Geometry check sheet. Reference: the model listing, model coordinates, mm. Face numbers are marked on the shaded views. A direction names the side the tool comes from. Round coordinates to 2 decimals unless told otherwise and drop trailing zeros. Write each loop counter-clockwise with the first axis right and the second up, starting at its lowest first coordinate (ties: lowest second). Pieces come first, ordered by that corner, then holes. Notation, with made-up numbers: (59, 5.5) - (79, 5.5) arc R24 cw to (79, 25.5) - close; hole circle Ø4 at (0.5, 8.5). An arc over 180 degrees is marked (long way). Return JSON: item names as keys, results as strings. Group by question number.
from build123d import *

# Parameters (mm, degrees)
SKETCH_2_R          = 1.5
EXTRUDE_1_DEPTH     = 27
SHELL_1_DEPTH       = 24
CUT_EXTRUDE_START   = -24
SKETCH_3_R          = 3
CUT_EXTRUDE_1_DEPTH = 24
SKETCH_5_W          = 20
SKETCH_5_H          = 6
CUT_EXTRUDE_3_DEPTH = 32
SKETCH_6_W          = 4
SKETCH_6_H          = 12
CUT_EXTRUDE_4_DEPTH = 32
SKETCH_7_W          = 10
SKETCH_7_H          = 8
CUT_EXTRUDE_5_DEPTH = 32
EXTRUDE_2_DEPTH     = 24
SKETCH_9_W          = 10
SKETCH_9_H          = 3
CUT_EXTRUDE_6_DEPTH = 24
SKETCH_10_R         = 1.35
CUT_EXTRUDE_7_DEPTH = 10
CUT_EXTRUDE_8_DEPTH = 10


# Read off the part's stored shape, not the designer's step: 抽壳1
with BuildPart() as part:
    # 草图2 → 凸台-拉伸1 (new body)
    with BuildSketch(Plane.XY):
        with BuildLine():
            Line((-76.5, 30.151923789), (-76.5, -30.151923789))
            ThreePointArc((-76.5, -30.151923789), (-77.380060021, -34.576284287), (-72.878679656, -34.871320344))
            Line((-72.878679656, -34.871320344), (-57.32, -50.43))
            Line((-57.32, -50.43), (57.32, -50.43))
            Line((57.32, -50.43), (72.878679656, -34.871320344))
            ThreePointArc((72.878679656, -34.871320344), (77.380060021, -34.576284287), (76.5, -30.151923789))
            Line((76.5, -30.151923789), (76.5, 30.151923789))
            ThreePointArc((76.5, 30.151923789), (77.593259199, 34.258312544), (73.483390382, 35.33841559))
            Line((73.483390382, 35.33841559), (40.238526366, 54.25))
            Line((40.238526366, 54.25), (-40.760907637, 54.25))
            Line((-40.760907637, 54.25), (-73.5, 35.348076211))
            ThreePointArc((-73.5, 35.348076211), (-77.598076211, 34.25), (-76.5, 30.151923789))
        make_face()
        with Locations((-75, 32.75)):
            Circle(SKETCH_2_R, mode=Mode.SUBTRACT)
        with Locations((75, 32.75)):
            Circle(SKETCH_2_R, mode=Mode.SUBTRACT)
        with Locations((75, -32.75)):
            Circle(SKETCH_2_R, mode=Mode.SUBTRACT)
        with Locations((-75, -32.75)):
            Circle(SKETCH_2_R, mode=Mode.SUBTRACT)
    extrude(amount=EXTRUDE_1_DEPTH)

    # 抽壳1 outline → 抽壳1 (cut)
    with BuildSketch(Plane.XY):
        with BuildLine():
            Line((-73.5, 28.507359313), (-73.5, -28.507359313))
            ThreePointArc((-73.5, -28.507359313), (-71.254879923, -30.255190266), (-70.506971411, -33.000387902))
            Line((-70.506971411, -33.000387902), (-56.077359313, -47.43))
            Line((-56.077359313, -47.43), (56.077359313, -47.43))
            Line((56.077359313, -47.43), (70.506971411, -33.000387902))
            ThreePointArc((70.506971411, -33.000387902), (71.254879923, -30.255190266), (73.5, -28.507359313))
            Line((73.5, -28.507359313), (73.5, 28.507359313))
            ThreePointArc((73.5, 28.507359313), (71.110106029, 30.48754008), (70.570593139, 33.543948905))
            Line((70.570593139, 33.543948905), (39.444948236, 51.25))
            Line((39.444948236, 51.25), (-39.95706006, 51.25))
            Line((-39.95706006, 51.25), (-70.575765386, 33.572282238))
            ThreePointArc((-70.575765386, 33.572282238), (-71.102885683, 30.5), (-73.5, 28.507359313))
        make_face()
    extrude(amount=SHELL_1_DEPTH, mode=Mode.SUBTRACT)

    # 草图3 → 切除-拉伸1 (cut)
    with BuildSketch(Plane.XY.offset(27).offset(CUT_EXTRUDE_START)):
        with Locations((75, 32.75)):
            Circle(SKETCH_3_R)
        with Locations((75, -32.75)):
            Circle(SKETCH_3_R)
        with Locations((-75, -32.75)):
            Circle(SKETCH_3_R)
        with Locations((-75, 32.75)):
            Circle(SKETCH_3_R)
    extrude(amount=CUT_EXTRUDE_1_DEPTH, mode=Mode.SUBTRACT)

    # 草图5 → 切除-拉伸3 (cut)
    with BuildSketch(Plane.XY.offset(27)):
        with Locations((20.7074416, -19.577067137)):
            Rectangle(SKETCH_5_W, SKETCH_5_H)
    extrude(amount=-CUT_EXTRUDE_3_DEPTH, mode=Mode.SUBTRACT)

    # 草图6 → 切除-拉伸4 (cut)
    with BuildSketch(Plane(origin=(76.5, 0, 0), x_dir=(0, 0, -1), z_dir=(1, 0, 0))):
        with Locations((-2, 20.977362477)):
            Rectangle(SKETCH_6_W, SKETCH_6_H)
    extrude(amount=-CUT_EXTRUDE_4_DEPTH, mode=Mode.SUBTRACT)

    # 草图7 → 切除-拉伸5 (cut)
    with BuildSketch(Plane(origin=(33.153284591, 58.280491682, 0), x_dir=(0.8692042501767389, -0.4944532045347601, 0), z_dir=(0.4944532045347601, 0.8692042501767389, 0))):
        with Locations((38.03253292, -4)):
            Rectangle(SKETCH_7_W, SKETCH_7_H)
    extrude(amount=-CUT_EXTRUDE_5_DEPTH, mode=Mode.SUBTRACT)

    # 草图8 → 凸台-拉伸2 (add)
    with BuildSketch(Plane.XY.offset(27)):
        Polygon((40.238526366, 54.25), (40.238526366, 62.25), (15.238526366, 62.25), (15.238526366, 54.25), (17.238526366, 54.25), (17.238526366, 60.25), (38.238526366, 60.25), (38.238526366, 54.25), align=None)
    extrude(amount=-EXTRUDE_2_DEPTH)

    # 草图9 → 切除-拉伸6 (cut)
    with BuildSketch(Plane(origin=(0, 54.25, 0), x_dir=(1, 0, 0), z_dir=(0, 1, 0))):
        with Locations((27.738526366, -1.5)):
            Rectangle(SKETCH_9_W, SKETCH_9_H)
    extrude(amount=-CUT_EXTRUDE_6_DEPTH, mode=Mode.SUBTRACT)

    # 草图10 → 切除-拉伸7 (cut)
    with BuildSketch(Plane.XZ.offset(50.43)):
        with Locations((-18.75, 20)):
            Circle(SKETCH_10_R)
        with Locations((18.75, 20)):
            Circle(SKETCH_10_R)
    extrude(amount=-CUT_EXTRUDE_7_DEPTH, mode=Mode.SUBTRACT)

    # 草图11 → 切除-拉伸8 (cut)
    with BuildSketch(Plane.XZ.offset(50.43)):
        Polygon((0, 3), (2, 3), (2, 0), (-2, 0), (-2, 3), align=None)
    extrude(amount=-CUT_EXTRUDE_8_DEPTH, mode=Mode.SUBTRACT)


solid = part.part
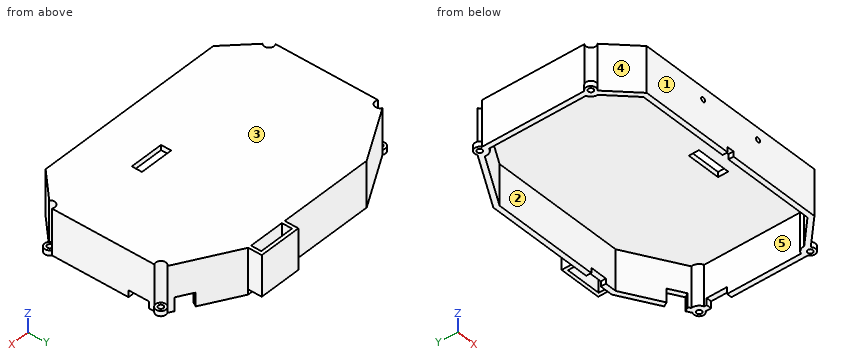
1. Section check B-B (x = 6). Enter the section's corners in (y, z), and give its area (3 significant figures).
2. Material ranges on line 1 along Y through (x, z) = (75, 1.7); line 2 along X through (y, z) = (-32.75, 2.15); line 3 along Y through (x, z) = (34.5, 18.5), recorded low to high.
3. Section check C-C (y = -11). Enter the section's corners in (x, z).
4. Depth check by flat-ended pin: pin 1 Ø2 at (x, z) = (-37, 23) entering from +Y; pin 2 Ø3 at (x, z) = (-45, 19) entering from +Y; pin 3 Ø2 at (x, y) = (57, -24) entering from -Z; pin 4 Ø5 at (x, y) = (-75, 32.75) entering from -Z. Enter the tip coordinate at first touch or a pass-through.
5. Section check A-A (z = 15.5). State how many separate pieces and enclosed holes the cut face has, and give its area (3 significant figures).
6. Tool access check on the marked faces 1 and 2. Record the directions out of +Z, -Z, +X, -X, +Y, -Y that give a thin tool (end or side, any length) a straight path to the whole face; none if there is none.
7. Mould release check, pull along Y, two halves, no side actions. Record for the marked faces 3, 4 and 5: pulls with the +Y half, pulls with the -Y half, needs draft (parallel to the pull), parting line crosses it, or undercut.
Result sheet:
{
 "1": {"outline": "(-50.43, 0) - (-47.43, 0) - (-47.43, 24) - (51.25, 24) - (51.25, 0) - (54.25, 0) - (54.25, 27) - (-50.43, 27) - close", "area": "458 mm²"},
 "2": {"line 1": "y = -35.75 to -34.25, -31.25 to 14.98, 26.98 to 31.25, 34.25 to 35.75", "line 2": "x = -78 to -76.5, -73.5 to -70.5, 70.5 to 73.5, 76.5 to 78", "line 3": "y = -50.43 to -47.43, 51.25 to 54.25, 60.25 to 62.25"},
 "3": {"outline": "(-76.5, 0) - (-73.5, 0) - (-73.5, 24) - (73.5, 24) - (73.5, 0) - (76.5, 0) - (76.5, 27) - (-76.5, 27) - close"},
 "4": {"pin 1": "stops at y = 54.25", "pin 2": "stops at y = 52.67", "pin 3": "stops at z = 24", "pin 4": "stops at z = 0"},
 "5": {"separate pieces": "1", "enclosed holes": "2", "area": "1,400 mm²"},
 "6": {"face 1": "+Z, -Z, +X, -X, -Y", "face 2": "-Z"},
 "7": {"face 3": "needs draft", "face 4": "pulls with the -Y half", "face 5": "undercut"}
}
